```python
from build123d import *

# Parameters (mm, degrees)
BOSS_EXTRUDE1_DEPTH = 22
CHAMFER1_SIZE       = 12
SKETCH2_R           = 2.25
CUT_EXTRUDE1_DEPTH  = 25
SKETCH2_4_R         = 4.5
SKETCH2_4_R_2       = 2.25
CUT_EXTRUDE2_DEPTH  = 21
CHAMFER2_SIZE       = 2
BOSS_EXTRUDE2_START = -22
BOSS_EXTRUDE2_DEPTH = 22
BOSS_EXTRUDE3_DEPTH = 4
BOSS_EXTRUDE4_START = -4
BOSS_EXTRUDE4_DEPTH = 4


with BuildPart() as part:
    # Sketch1 → Boss-Extrude1 (new body)
    with BuildSketch(Plane(origin=(0, 0, 0), x_dir=(1, 0, 0), z_dir=(0, 0, -1))):
        with BuildLine():
            Line((-38.985549133, -2.028901734), (-48.985549133, -2.028901734))
            Line((-48.985549133, -2.028901734), (-48.985549133, 22.971098266))
            Line((-48.985549133, 22.971098266), (6.014450867, 22.971098266))
            Line((6.014450867, 22.971098266), (6.014450867, -2.028901734))
            Line((6.014450867, -2.028901734), (-3.985549133, -2.028901734))
            ThreePointArc((-3.985549133, -2.028901734), (-21.485549133, 15.471098266), (-38.985549133, -2.028901734))
        make_face()
    extrude(amount=BOSS_EXTRUDE1_DEPTH)

    # Chamfer1
    chamfer1_edges = [part.edges().sort_by_distance(p)[0] for p in [
        (-48.985549133, -22.971098266, -11),
        (6.014450867, -22.971098266, -11),
    ]]
    chamfer(chamfer1_edges, length=CHAMFER1_SIZE)

    # Sketch2 → Cut-Extrude1 (cut)
    with BuildSketch(Plane(origin=(0, -22.971098266, 0), x_dir=(-1, 0, 0), z_dir=(0, -1, 0))):
        with Locations(Location((43.985549133, 11, 0), (0, 0, 180))):
            Circle(SKETCH2_R)
        with Locations((-1.014450867, 11)):
            Circle(SKETCH2_R)
    extrude(amount=-CUT_EXTRUDE1_DEPTH, mode=Mode.SUBTRACT)

    # Sketch2<4> → Cut-Extrude2 (cut)
    # profile 1 of 2: a face of its own
    with BuildSketch(Plane(origin=(0, -22.971098266, 0), x_dir=(-1, 0, 0), z_dir=(0, -1, 0))):
        with Locations(Location((43.985549133, 11, 0), (0, 0, 180))):
            Circle(SKETCH2_4_R)
        with Locations(Location((43.985549133, 11, 0), (0, 0, 180))):
            Circle(SKETCH2_4_R_2, mode=Mode.SUBTRACT)
    # profile 2 of 2: a face of its own
    with BuildSketch(Plane(origin=(0, -22.971098266, 0), x_dir=(-1, 0, 0), z_dir=(0, -1, 0))):
        with Locations((-1.014450867, 11)):
            Circle(SKETCH2_4_R)
        with Locations(Location((-1.014450867, 11, 0), (0, 0, 180))):
            Circle(SKETCH2_4_R_2, mode=Mode.SUBTRACT)
    extrude(amount=-CUT_EXTRUDE2_DEPTH, mode=Mode.SUBTRACT)

    # Chamfer2
    chamfer2_edges = [part.edges().sort_by_distance(p)[0] for p in [
        (6.014450867, -4.471098266, -22),
        (-21.485549133, -22.971098266, 0),
        (-21.485549133, -22.971098266, -22),
        (-48.985549133, -4.471098266, 0),
        (-42.985549133, -16.971098266, 0),
        (0.014450867, -16.971098266, 0),
        (-48.985549133, -4.471098266, -22),
        (-42.985549133, -16.971098266, -22),
        (0.014450867, -16.971098266, -22),
        (6.014450867, -4.471098266, 0),
    ]]
    chamfer(chamfer2_edges, length=CHAMFER2_SIZE)

    # Sketch3 → Boss-Extrude2 (add)
    with BuildSketch(Plane(origin=(0, 0, -22), x_dir=(-1, 0, 0), z_dir=(0, 0, -1)).offset(BOSS_EXTRUDE2_START)):
        with BuildLine():
            Line((3.985549133, 2.028901734), (10.485549133, 2.028901734))
            ThreePointArc((10.485549133, 2.028901734), (21.485549133, -8.971098266), (32.485549133, 2.028901734))
            Line((32.485549133, 2.028901734), (38.985549133, 2.028901734))
            ThreePointArc((38.985549133, 2.028901734), (21.485549133, -15.471098266), (3.985549133, 2.028901734))
        make_face()
    extrude(amount=BOSS_EXTRUDE2_DEPTH)

    # Sketch4 → Boss-Extrude3 (add)
    with BuildSketch(Plane.XY):
        with BuildLine():
            Line((-32.485549133, 2.028901734), (-28.985549133, 2.028901734))
            ThreePointArc((-28.985549133, 2.028901734), (-21.485549133, -5.471098266), (-13.985549133, 2.028901734))
            Line((-13.985549133, 2.028901734), (-10.485549133, 2.028901734))
            ThreePointArc((-10.485549133, 2.028901734), (-21.485549133, -8.971098266), (-32.485549133, 2.028901734))
        make_face()
    extrude(amount=-BOSS_EXTRUDE3_DEPTH)

    # Sketch5 → Boss-Extrude4 (add)
    with BuildSketch(Plane(origin=(0, 0, -22), x_dir=(-1, 0, 0), z_dir=(0, 0, -1)).offset(BOSS_EXTRUDE4_START)):
        with BuildLine():
            Line((10.485549133, 2.028901734), (13.985549133, 2.028901734))
            ThreePointArc((13.985549133, 2.028901734), (21.485549133, -5.471098266), (28.985549133, 2.028901734))
            Line((28.985549133, 2.028901734), (32.485549133, 2.028901734))
            ThreePointArc((32.485549133, 2.028901734), (21.485549133, -8.971098266), (10.485549133, 2.028901734))
        make_face()
    extrude(amount=BOSS_EXTRUDE4_DEPTH)


solid = part.part
```
Design review of the part built by this model. Coordinates are the model's own, in mm. A direction names the side the tool comes from. Coordinates: 2 decimals unless noted, no trailing zeros. Order: outer loops, then holes, each group sorted by start corner. A loop starts at its lowest first (then second) coordinate and runs counter-clockwise, first axis right, second up. Notation, with made-up numbers: (-14, 19) -> (-1, 19) arc R3 cw to (-1, 24) -> close; hole circle Ø1 at (77.25, 10.25). An arc over 180 degrees is marked (long way). One line per item, written item: value. Start each with the question number.
Q1. Take a section at C-C, the plane x = 0.5. State the section outline as (y, z) points, then the cut area to 3 significant figures.
Q2. Take a section at A-A, the plane y = -0.5. State the section outline as (x, z) points, then the cut area to 3 significant figures.
Q3. Tool access review of faces 1 (the flat face through (-22, -6, -18)), 2 (the flat face through (-42.37, -16.19, -20.99)), 3 (the flat face through (-42, -1.971, -13)): name each direction out of +Z, -Z, +X, -X, +Y, -Y from which nothing blocks a thin tool from reaching the whole face with its end or side.
Q4. Insertion check: pin 1 Ø12 at (x, z) = (-0.5, -18.5) entering from -Y; pin 2 Ø10 at (x, z) = (-45, -9) entering from -Y; pin 3 Ø4.5 at (x, z) = (0.5, -10) entering from -Y; pin 4 Ø1 at (y, z) = (-15.5, -10.5) entering from +X. Each pin has a flat end and moves straight along its axis. Give the tip position at first contact, or say it passes through.
Q5. Take a section at D-D, the plane y = -9.5. State the section outline as (x, z) points.
Q6. Take a section at B-B, the plane z = -16.75. State the section outline as (x, y) points, then the cut area to 3 significant figures.
Q7. For probe 1 along X at (y, z) = (-10, -11.25); probe 2 along Z at (x, y) = (-13, -4.5); probe 3 along X at (y, z) = (-3, -11), list the stretches that pass through material, from the lowest coordinate up.
Q8. Mouldability with a two-part tool opening along X and no side actions: class faces 4 (the cylindrical face through (-21.32, -5.47, -19.97)), 5 (the flat face through (-4, 2.029, -11)), 6 (the flat face through (5.028, -4.562, -20.986)) as pulls with the +X half, pulls with the -X half, needs draft (parallel to the pull), parting line crosses it, or undercut.
Values follow:
1. outline: (-16.49, -20) -> (-13.66, -22) -> (2.03, -22) -> (2.03, -13.19) -> (-1.97, -13.19) -> (-1.97, -15.47) -> (-16.49, -15.47) -> close; (-16.49, -6.53) -> (-1.97, -6.53) -> (-1.97, -8.81) -> (2.03, -8.81) -> (2.03, 0) -> (-13.66, 0) -> (-16.49, -2) -> close
1. area: 254 mm2
2. outline: (-48.99, -20) -> (-46.99, -22) -> (-28.55, -22) -> (-28.55, -18) -> (-32.19, -18) -> (-32.19, -4) -> (-28.55, -4) -> (-28.55, 0) -> (-46.99, 0) -> (-48.99, -2) -> close; (-14.42, -22) -> (4.01, -22) -> (6.01, -20) -> (6.01, -2) -> (4.01, 0) -> (-14.42, 0) -> (-14.42, -4) -> (-10.78, -4) -> (-10.78, -18) -> (-14.42, -18) -> close; hole circle Ø4.5 at (-43.99, -11); hole circle Ø4.5 at (1.01, -11)
2. area: 757 mm2
3. face 1: +Y
3. face 2: -Z, -X, -Y
3. face 3: -Y
4. pin 1: stops at y = -22.97
4. pin 2: stops at y = -19.96
4. pin 3: stops at y = -1.97
4. pin 4: stops at x = -3.37
5. outline: (-48.99, -20) -> (-46.99, -22) -> (4.01, -22) -> (6.01, -20) -> (6.01, -2) -> (4.01, 0) -> (-46.99, 0) -> (-48.99, -2) -> close; hole circle Ø9 at (-43.99, -11); hole circle Ø9 at (1.01, -11)
6. outline: (-48.99, -10.97) -> (-36.99, -22.97) -> (-5.99, -22.97) -> (6.01, -10.97) -> (6.01, 2.03) -> (-10.49, 2.03) arc R11 cw to (-32.49, 2.03) -> (-48.99, 2.03) -> close
6. area: 1,040 mm2
7. probe 1: x = -48.99 to -48.48, -39.49 to -3.48, 5.51 to 6.01
7. probe 2: z = -22 to -18, -4 to 0
7. probe 3: x = -48.99 to -48.49, -39.49 to -31.27, -11.7 to -3.49, 5.51 to 6.01
8. face 4: undercut
8. face 5: needs draft
8. face 6: pulls with the +X half
